from build123d import *

# Parameters (mm, degrees)
SKETCH1_R                = 37.973
BOSS_EXTRUDE1_DEPTH      = 1.5875
H_0_266_DIAMETER_HOLE1_D = 6.7564
H_0_266_DIAMETER_HOLE2_D = 6.7564


with BuildPart() as part:
    # Sketch1 → Boss-Extrude1 (new, symmetric)
    with BuildSketch(Plane(origin=(0, 0, 0), x_dir=(1, 0, 0), z_dir=(0, 1, 0))):
        with Locations(Location((0, 0, 0), (0, 0, 270))):
            Circle(SKETCH1_R)
    extrude(amount=BOSS_EXTRUDE1_DEPTH, both=True)

    # H (0.266) Diameter Hole1 (through all)
    with Locations(Plane(origin=(0, 1.5875, 0), x_dir=(1, 0, 0), z_dir=(0, 1, 0))):
        with Locations((-28.575, 0), (28.575, 0)):
            Hole(H_0_266_DIAMETER_HOLE1_D / 2)

    # H (0.266) Diameter Hole2 (through all)
    with Locations(Plane(origin=(0, 1.5875, 0), x_dir=(1, 0, 0), z_dir=(0, 1, 0))):
        with Locations((0, 0)):
            Hole(H_0_266_DIAMETER_HOLE2_D / 2)


solid = part.part
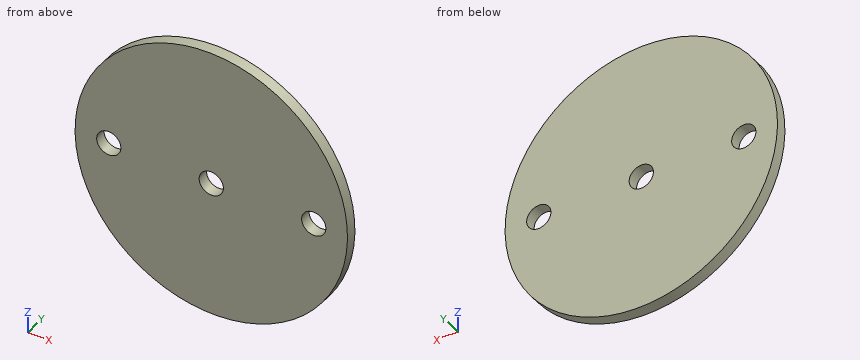
Can you work these out from the model? Positions are in its coordinate system, mm. Coordinates: 2 decimals unless noted, no trailing zeros. Write each loop counter-clockwise with the first axis right and the second up, starting at its lowest first coordinate (ties: lowest second). Pieces come first, ordered by that corner, then holes. Notation, with made-up numbers: (-6.5, 60) -> (49.5, 60) arc R17 ccw to (49.5, 85) -> close; hole circle Ø11 at (76.5, 82). An arc over 180 degrees is marked (long way). Write item = value, one per line.
(1) Imagine slicing it at A-A (x = 0). Please give me the cut outline in (y, z).
Verdict:
outline = (-1.59, -37.97) -> (1.59, -37.97) -> (1.59, -3.38) -> (-1.59, -3.38) -> close; (-1.59, 3.38) -> (1.59, 3.38) -> (1.59, 37.97) -> (-1.59, 37.97) -> close
(2) Imagine slicing it at B-B (z = 0). Please give me the cut outline in (x, y), and give its area (3 significant figures).
Verdict:
outline = (-37.97, -1.59) -> (-31.95, -1.59) -> (-31.95, 1.59) -> (-37.97, 1.59) -> close; (-25.2, -1.59) -> (-3.38, -1.59) -> (-3.38, 1.59) -> (-25.2, 1.59) -> close; (3.38, -1.59) -> (25.2, -1.59) -> (25.2, 1.59) -> (3.38, 1.59) -> close; (31.95, -1.59) -> (37.97, -1.59) -> (37.97, 1.59) -> (31.95, 1.59) -> close
area = 177 mm^2
(3) If I drill on probe 1 along Z at (x, y) = (27.5, 1.2); probe 2 along X at (y, z) = (-0.1, 3); probe 3 along Z at (x, y) = (29, 0.05), over which ranges is the centre line in solid material (lowest first)?
Verdict:
probe_1 = -26.19 to -3.2, 3.2 to 26.19
probe_2 = -37.85 to -30.13, -27.02 to -1.55, 1.55 to 27.02, 30.13 to 37.85
probe_3 = -24.51 to -3.35, 3.35 to 24.51
(4) Imagine slicing it at D-D (z = 26). Please give me the cut outline in (x, y), and give its area (3 significant figures).
Verdict:
outline = (-27.68, -1.59) -> (27.68, -1.59) -> (27.68, 1.59) -> (-27.68, 1.59) -> close
area = 176 mm^2
(5) Imagine slicing it at C-C (y = -0.1). Please give me the cut outline in (x, z) (3 decimals).
Verdict:
outline = circle Ø75.946 at (0, 0); hole circle Ø6.756 at (-28.575, 0); hole circle Ø6.756 at (0, 0); hole circle Ø6.756 at (28.575, 0)
